Geometry check sheet. Reference: drawing and pictorial views, mm from the part's lowest x, y, z. Coordinates: 2 decimals unless noted, no trailing zeros. Write each loop counter-clockwise with the first axis right and the second up, starting at its lowest first coordinate (ties: lowest second). Pieces come first, ordered by that corner, then holes. Notation, with made-up numbers: (21, 1) -> (57, 1) arc R26 cw to (57, 37) -> close; hole circle Ø3 at (-2, 17.5). An arc over 180 degrees is marked (long way). Answer in a Markdown table with one row per item.
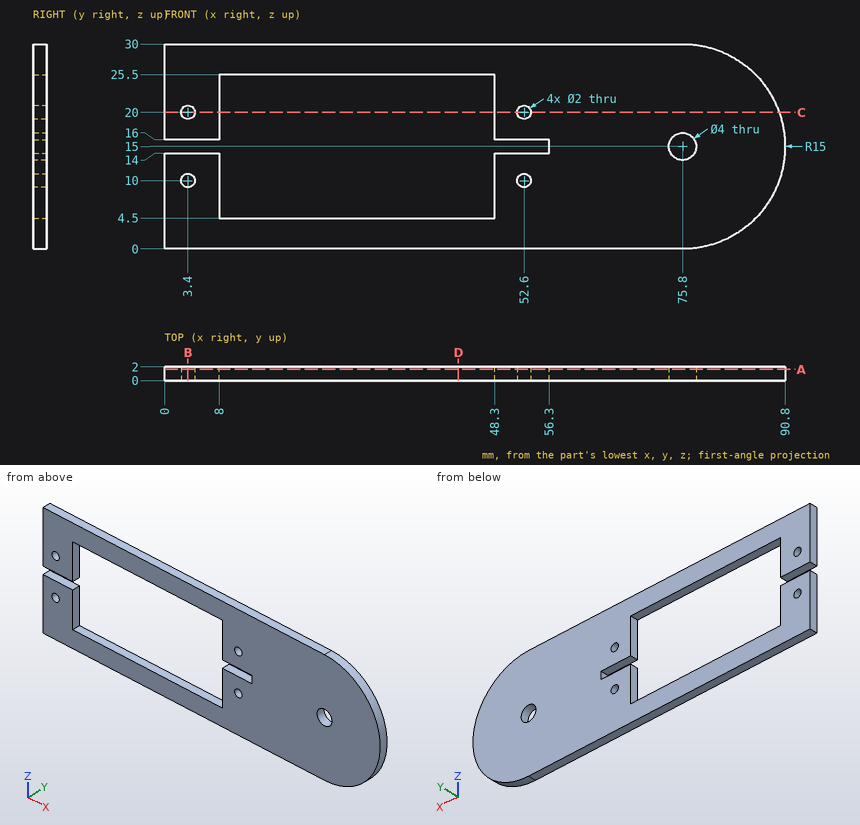
1. Section check B-B, the plane x = 3.4. Record the boundary of the cut face in (y, z), plus the area to 3 significant figures.
Geometry says:
| item | result |
|---|---|
| outline | (0, 0) -> (2, 0) -> (2, 9) -> (0, 9) -> close; (0, 11) -> (2, 11) -> (2, 14) -> (0, 14) -> close; (0, 16) -> (2, 16) -> (2, 19) -> (0, 19) -> close; (0, 21) -> (2, 21) -> (2, 30) -> (0, 30) -> close |
| area | 48.0 mm^2 |
2. Section check A-A, the plane y = 1.65. Record the boundary of the cut face in (x, z), plus the area to 3 significant figures.
Geometry says:
| item | result |
|---|---|
| outline | (0, 0) -> (75.8, 0) arc R15 ccw to (75.8, 30) -> (0, 30) -> (0, 16) -> (8, 16) -> (8, 25.5) -> (48.3, 25.5) -> (48.3, 16) -> (56.3, 16) -> (56.3, 14) -> (48.3, 14) -> (48.3, 4.5) -> (8, 4.5) -> (8, 14) -> (0, 14) -> close; hole circle Ø2 at (3.4, 10); hole circle Ø2 at (3.4, 20); hole circle Ø2 at (52.6, 10); hole circle Ø2 at (52.6, 20); hole circle Ø4 at (75.8, 15) |
| area | 1,720 mm^2 |
3. Depth check by flat-ended pin: P1, Ø1.8, axis at x = 52.6, z = 20, coming from the -Y side; P2, Ø5, axis at x = 75.8, z = 15, coming from the -Y side. Enter the tip coordinate at first touch or a pass-through.
Geometry says:
| item | result |
|---|---|
| P1 | through |
| P2 | y = 0 |
4. Section check D-D, the plane x = 43. Record the boundary of the cut face in (y, z).
Geometry says:
| item | result |
|---|---|
| outline | (0, 0) -> (2, 0) -> (2, 4.5) -> (0, 4.5) -> close; (0, 25.5) -> (2, 25.5) -> (2, 30) -> (0, 30) -> close |
5. Section check C-C, the plane z = 20. Record the boundary of the cut face in (x, y).
Geometry says:
| item | result |
|---|---|
| outline | (0, 0) -> (2.4, 0) -> (2.4, 2) -> (0, 2) -> close; (4.4, 0) -> (8, 0) -> (8, 2) -> (4.4, 2) -> close; (48.3, 0) -> (51.6, 0) -> (51.6, 2) -> (48.3, 2) -> close; (53.6, 0) -> (89.94, 0) -> (89.94, 2) -> (53.6, 2) -> close |
6. Thickness scan on line 1 (Z direction, x = 9.5, y = 1.05); line 2 (Z direction, x = 75.8, y = 1.3); line 3 (X direction, y = 1.1, z = 10). Record the ranges inside material, lowest first. Write a range as from..to.
Geometry says:
| item | result |
|---|---|
| line 1 | 0..4.5, 25.5..30 |
| line 2 | 0..13, 17..30 |
| line 3 | 0..2.4, 4.4..8, 48.3..51.6, 53.6..89.94 |
